```python
from build123d import *

# Parameters (mm, degrees)
SKETCH1_R             = 14.2875
BOSS_EXTRUDE1_DEPTH   = 6.35
SKETCH2_R             = 7.3025
BOSS_EXTRUDE2_DEPTH   = 20.6375
CUT_EXTRUDE1_REACH    = 35.713
SKETCH3_R             = 3.4925
F_8_CLEARANCE_HOLE1_D = 4.4958


with BuildPart() as part:
    # Sketch1 → Boss-Extrude1 (new body)
    with BuildSketch(Plane(origin=(0, 0, 0), x_dir=(1, 0, 0), z_dir=(0, 1, 0))):
        with Locations(Location((0, 0, 0), (0, 0, 270))):
            Circle(SKETCH1_R)
    extrude(amount=BOSS_EXTRUDE1_DEPTH)

    # Sketch2 → Boss-Extrude2 (add)
    with BuildSketch(Plane(origin=(0, 6.35, 0), x_dir=(1, 0, 0), z_dir=(0, 1, 0))):
        with Locations(Location((0, 0, 0), (0, 0, 270))):
            Circle(SKETCH2_R)
    extrude(amount=BOSS_EXTRUDE2_DEPTH)

    # Sketch3 → Cut-Extrude1 (cut, up to next)
    with BuildSketch(Plane.XZ, mode=Mode.PRIVATE) as cut_extrude1_sk1:
        with Locations(Location((0, 0, 0), (0, 0, 270))):
            Circle(SKETCH3_R)
    cut_extrude1_tool1 = extrude(cut_extrude1_sk1.sketch, amount=-CUT_EXTRUDE1_REACH, mode=Mode.PRIVATE) & part.part
    add(cut_extrude1_tool1.solids().sort_by_distance((0, 0, 0))[0], mode=Mode.SUBTRACT)

    # #8 Clearance Hole1 (through all)
    with Locations(Plane(origin=(0, 0, 0), x_dir=(-1, 0, 0), z_dir=(0, -1, 0))):
        with Locations((-5.55625, 9.6237073), (11.1125, 0), (-5.55625, -9.6237073)):
            Hole(F_8_CLEARANCE_HOLE1_D / 2)


solid = part.part
```
CAD build for the part. Positions are in the model's coordinates, mm. Round coordinates to 2 decimals unless told otherwise and drop trailing zeros. Loops run counter-clockwise (first coordinate to the right, second up) from the corner with the lowest first, then second, coordinate; pieces in that order, holes last. Notation, with made-up numbers: (-16, 84) - (28, 84) arc R23 cw to (28, 99) - close; hole circle Ø7 at (44, 5). An arc over 180 degrees is marked (long way). Return JSON: item names as keys, results as strings. Group by question number.
Q1. Band-saw the part on D-D on y = 20. Give the cut face in (x, z) (1 decimal), plus the area to 3 significant figures.
Q2. Band-saw the part on C-C on z = -8.5. Give the cut face in (x, y).
Q3. Two-plate mould, pull along X, no slides. Class faces 1 (the face through (-13.36, 3.22, -0.1)), 2 (the face through (6.157, 16.524, 3.926)), 3 (the face through (7, 6.35, -3)): +X half, -X half, draft (parallel to the pull), parting line (faces both ways), or undercut.
Q4. Flat gauge pins, fed straight in: pin 1 Ø1 at (y, z) = (6.5, 9.5) entering from -X; pin 2 Ø8 at (x, y) = (-8.5, 7) entering from +Z; pin 3 Ø8 at (y, z) = (16, 4.5) entering from -X. Where does each tip first touch, or does it go through?
Q5. Drill centre lines: line 1 along X through (y, z) = (9.5, 0); line 2 along Y through (x, z) = (-4.75, -12.25); line 3 along X through (y, z) = (1.75, -7.75). Where is each one in solid material? Low to high. Write a range as [from, to].
Q6. Band-saw the part on B-B on z = 0. Give the cut face in (x, y).
Q7. Band-saw the part on A-A on x = 0. Give the cut face in (y, z).
Solutions:
{
 "1": {"outline": "circle Ø14.6 at (0, 0); hole circle Ø7 at (0, 0)", "area": "129 mm^2"},
 "2": {"outline": "(-11.48, 0) - (3.61, 0) - (3.61, 6.35) - (-11.48, 6.35) - close; (7.5, 0) - (11.48, 0) - (11.48, 6.35) - (7.5, 6.35) - close"},
 "3": {"face 1": "undercut", "face 2": "parting line", "face 3": "draft"},
 "4": {"pin 1": "stops at x = -11.08", "pin 2": "stops at z = 13.54", "pin 3": "stops at x = -7.29"},
 "5": {"line 1": "x = [-7.3, -3.49], [3.49, 7.3]", "line 2": "y = [0, 6.35]", "line 3": "x = [-12, 4.31], [6.8, 12]"},
 "6": {"outline": "(-14.29, 0) - (-13.36, 0) - (-13.36, 6.35) - (-14.29, 6.35) - close; (-8.86, 0) - (-3.49, 0) - (-3.49, 26.99) - (-7.3, 26.99) - (-7.3, 6.35) - (-8.86, 6.35) - close; (3.49, 0) - (14.29, 0) - (14.29, 6.35) - (7.3, 6.35) - (7.3, 26.99) - (3.49, 26.99) - close"},
 "7": {"outline": "(0, -14.29) - (6.35, -14.29) - (6.35, -7.3) - (26.99, -7.3) - (26.99, -3.49) - (0, -3.49) - close; (0, 3.49) - (26.99, 3.49) - (26.99, 7.3) - (6.35, 7.3) - (6.35, 14.29) - (0, 14.29) - close"}
}
